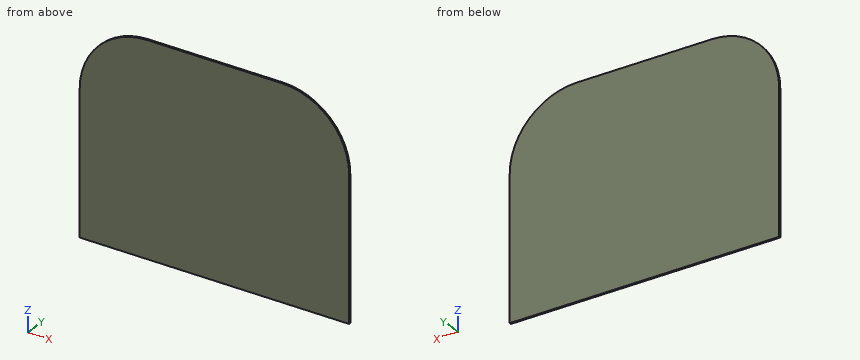
Solid Edge part; units mm, degrees
sketch "Sketch1" plane through (0, 0, 0) normal (0, -1, 0) x (1, 0, 0)
  line L0 (240, 250.22) -> (80, 250.22)
  arc A0 (80, 250.22) -> (0, 170.22) centre (80, 170.22) ccw
  line L1 (0, 170.22) -> (0, 0)
  line L2 (0, 0) -> (320, 0)
  line L3 (320, 0) -> (320, 170.22)
  arc A1 (320, 170.22) -> (240, 250.22) centre (240, 170.22) ccw
extrude "Protrusion1" add sketch "Sketch1" against normal blind 2
properties material "Aluminum, 1060"
Can you work these out from the model? Positions are in its coordinate system, mm. Coordinates: 2 decimals unless noted, no trailing zeros. Loops run counter-clockwise (first coordinate to the right, second up) from the corner with the lowest first, then second, coordinate; pieces in that order, holes last. Notation, with made-up numbers: (62, 1) - (95, 1) arc R29 ccw to (95, 25) - close; hole circle Ø2 at (25, 11). An arc over 180 degrees is marked (long way). Put each result on its own line as item: value. Start each with the question number.
Item 1: Suppose I cut it at C-C (z = 208.5). Please give me the cut outline in (x, y).
Item 2: Suppose I cut it at A-A (y = 0.8). Please give me the cut outline in (x, z), and give its area (3 significant figures).
Item 3: Suppose I cut it at B-B (x = 283.5). Please give me the cut outline in (y, z).
Item 4: If I drill on line 1 along Z through (x, y) = (303, 1.2); line 2 along Z through (x, y) = (29.5, 0.85); line 3 along X through (y, z) = (0.35, 228), over which ranges is the centre line in solid material (lowest first)?
Item 5: For pin 1 (1 mm diameter, centred on y = 1, z = 188, fed in from +X), with a flat end and sliding along its axis, tell me the tip position at first contact or that it passes through.
Here are the results:
1. outline: (9.75, 0) - (310.25, 0) - (310.25, 2) - (9.75, 2) - close
2. outline: (0, 0) - (320, 0) - (320, 170.22) arc R80 ccw to (240, 250.22) - (80, 250.22) arc R80 ccw to (0, 170.22) - close
2. area: 77,300 mm²
3. outline: (0, 0) - (2, 0) - (2, 237.36) - (0, 237.36) - close
4. line 1: 0 to 219.53
4. line 2: 0 to 232.27
4. line 3: 24.67 to 295.33
5. pin 1: x = 318.11
